For this review, take the finished solid that the model builds, in its own axes (mm). A direction names the side the tool comes from. Give positions to 0.01 mm unless a question says otherwise; leave off trailing zeros. Loops run counter-clockwise (first coordinate to the right, second up) from the corner with the lowest first, then second, coordinate; pieces in that order, holes last. Notation, with made-up numbers: (62, 76) - (119, 76) arc R25 ccw to (119, 92) - close; hole circle Ø11 at (10, 27). An arc over 180 degrees is marked (long way). Answer as CSV lines item,"result".
from build123d import *

# Parameters (mm, degrees)
BOSS_EXTRUDE1_DEPTH = 4


with BuildPart() as part:
    # Sketch1 → Boss-Extrude1 (new body)
    with BuildSketch(Plane.XY):
        with BuildLine():
            Line((0, 0), (10, 0))
            Line((10, 0), (10, 4))
            Line((10, 4), (14, 4))
            Line((14, 4), (14, 8))
            Line((14, 8), (10, 8))
            Line((10, 8), (10, 22))
            ThreePointArc((10, 22), (5, 27), (0, 22))
            Line((0, 22), (0, 8))
            Line((0, 8), (-4, 8))
            Line((-4, 8), (-4, 4))
            Line((-4, 4), (0, 4))
            Line((0, 4), (0, 0))
        make_face()
        Polygon((3.5, 17.401923789), (6.5, 17.401923789), (8, 20), (6.5, 22.598076211), (3.5, 22.598076211), (2, 20), align=None, mode=Mode.SUBTRACT)
        Polygon((8, 10.5), (6.5, 13.098076211), (3.5, 13.098076211), (2, 10.5), (3.5, 7.901923789), (6.5, 7.901923789), align=None, mode=Mode.SUBTRACT)
    extrude(amount=BOSS_EXTRUDE1_DEPTH)


solid = part.part
1) Wall thickness on line 1 (Y direction, x = 3.75, z = 1.5); line 2 (Y direction, x = 4, z = 0.25); line 3 (Y direction, x = -2, z = 2.95): over which ranges is each line inside the solid? List them lowest first. Write a range as from..to.
From the geometry:
line 1,"y = 0..7.9, 13.1..17.4, 22.6..26.84"
line 2,"y = 0..7.9, 13.1..17.4, 22.6..26.9"
line 3,"y = 4..8"
2) Insertion check: P1, Ø2, axis at y = 1.5, z = 1, coming from the -X side; P2, Ø5, axis at x = 3, y = 19.5, coming from the +Z side; P3, Ø1.2, axis at x = 12.5, z = 1.5, coming from the +Y side; P4, Ø1.2, axis at y = 3, z = 2.5, coming from the +X side. Each pin has a flat end and moves straight along its axis. Give the tip position at first contact, or say it passes through.
From the geometry:
P1,"stops at x = 0"
P2,"stops at z = 4"
P3,"stops at y = 8"
P4,"stops at x = 10"
3) Consider section C-C on y = 10. Write out the cut boundary in (x, z), and give its area (3 significant figures).
From the geometry:
outline,"(0, 0) - (2.29, 0) - (2.29, 4) - (0, 4) - close; (7.71, 0) - (10, 0) - (10, 4) - (7.71, 4) - close"
area,"18.3 mm^2"
4) Machinability: for faces 4 (the flat face through (0, 2, 2)), 5 (the flat face through (12, 4, 2)), 6 (the flat face through (5, 7.902, 2)), 7 (the flat face through (12, 8, 2)), 8 (the flat face through (-2, 8, 2)), which of the approach directions +Z, -Z, +X, -X, +Y, -Y give a long, thin tool a straight path to every point of the face, cutting with its end or side? Answer none if there is none.
From the geometry:
face 4,"+Z, -Z, -X, -Y"
face 5,"+Z, -Z, +X, -Y"
face 6,"+Z, -Z"
face 7,"+Z, -Z, +X, +Y"
face 8,"+Z, -Z, -X, +Y"
5) Consider section B-B on z = 2.4. Write out the cut boundary in (x, y), and give its area (3 significant figures).
From the geometry:
outline,"(-4, 4) - (0, 4) - (0, 0) - (10, 0) - (10, 4) - (14, 4) - (14, 8) - (10, 8) - (10, 22) arc R5 ccw to (0, 22) - (0, 8) - (-4, 8) - close; hole (2, 10.5) - (3.5, 7.9) - (6.5, 7.9) - (8, 10.5) - (6.5, 13.1) - (3.5, 13.1) - close; hole (2, 20) - (3.5, 17.4) - (6.5, 17.4) - (8, 20) - (6.5, 22.6) - (3.5, 22.6) - close"
area,"245 mm^2"
6) Consider section D-D on x = -0.75. Write out the cut boundary in (y, z), and give its area (3 significant figures).
From the geometry:
outline,"(4, 0) - (8, 0) - (8, 4) - (4, 4) - close"
area,"16.0 mm^2"
7) Consider section A-A on x = 5. Write out the cut boundary in (y, z).
From the geometry:
outline,"(0, 0) - (7.9, 0) - (7.9, 4) - (0, 4) - close; (13.1, 0) - (17.4, 0) - (17.4, 4) - (13.1, 4) - close; (22.6, 0) - (27, 0) - (27, 4) - (22.6, 4) - close"
8) Draft analysis for pull direction X (two halves, no side actions). For faces 1 (the flat face through (7.24, 18.68, 1.97)), 2 (the cylindrical face through (5, 27, 2)), 3 (the flat face through (-4, 6, 2)), state which applies: pulls with the +X half, pulls with the -X half, needs draft (parallel to the pull), parting line crosses it, or undercut.
From the geometry:
face 1,"undercut"
face 2,"parting line crosses it"
face 3,"pulls with the -X half"
